Part print with two shaded views. Sizes in mm from the minimum x, y, z corner. A direction names the side the tool comes from. Give positions to 0.01 mm unless a question says otherwise; leave off trailing zeros. Write each loop counter-clockwise with the first axis right and the second up, starting at its lowest first coordinate (ties: lowest second). Pieces come first, ordered by that corner, then holes. Notation, with made-up numbers: (77.25, 6) - (120.25, 6) arc R28 cw to (120.25, 25) - close; hole circle Ø2 at (-39, 18). An arc over 180 degrees is marked (long way). Answer as a JSON object with one key per item and string values. Group by question number.
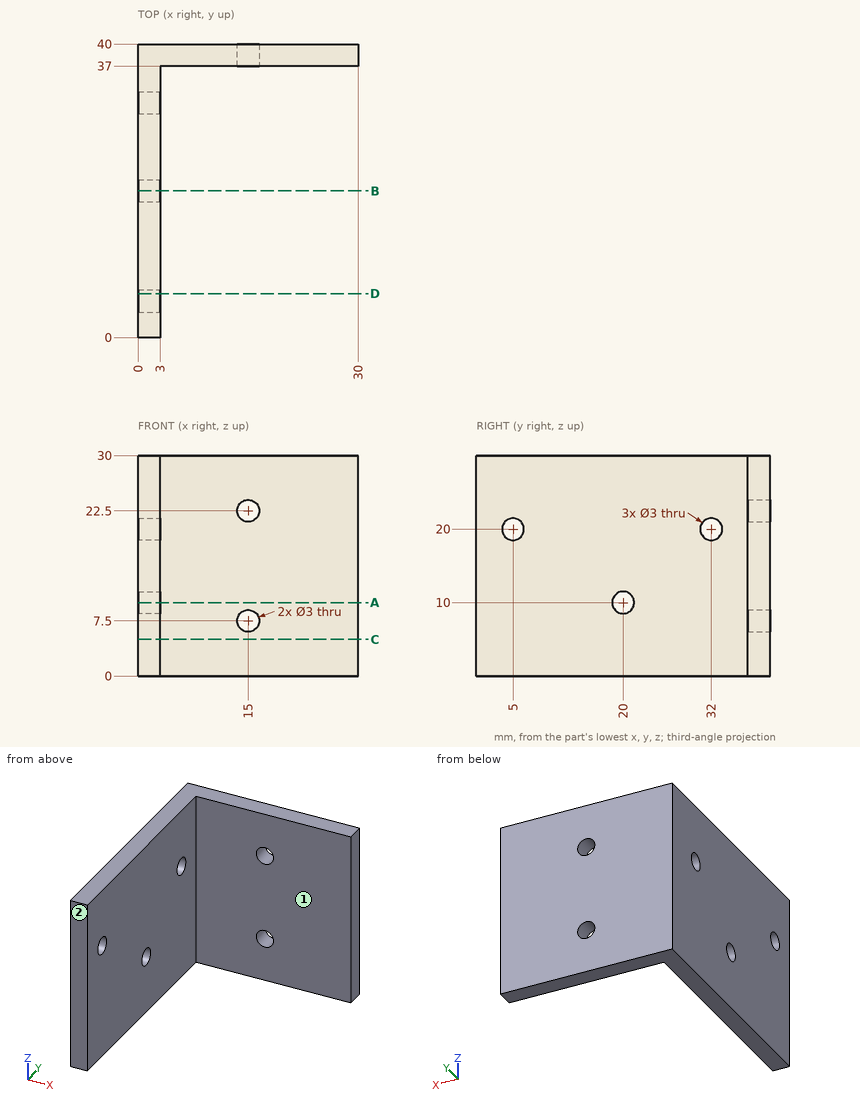
1) Drill centre lines: line 1 along Z through (x, y) = (15, 39.2); line 2 along Y through (x, z) = (2.35, 20); line 3 along X through (y, z) = (38.5, 22.5). Where is each one in solid material? Low to high. Write a range as from..to.
2) Drop flat-ended pins along their axis: P1, Ø1.8, axis at x = 15, z = 7.5, coming from the +Y side; P2, Ø1.5, axis at x = 17.5, z = 7.5, coming from the -Y side; P3, Ø1, axis at y = 26.5, z = 10, coming from the +X side. Give the stop position or say it passes through.
3) Saw through at A-A (z = 10). List the corners of the cut face in (x, y), and give its area (3 significant figures).
4) Which spindle directions (+Z, -Z, +X, -X, +Y, -Y) get a long thin tool onto all of the face, cutting with end or side? Do the marked faces 1 and 2. Say none if no direction does.
5) Saw through at D-D (y = 6). List the corners of the cut face in (x, z), and give its area (3 significant figures).
6) Saw through at C-C (z = 5). List the corners of the cut face in (x, y).
7) Saw through at B-B (y = 20). List the corners of the cut face in (x, z).
Checks:
{
 "1": {"line 1": "0..6, 9..21, 24..30", "line 2": "0..3.5, 6.5..30.5, 33.5..40", "line 3": "0..13.5, 16.5..30"},
 "2": {"P1": "through", "P2": "y = 37", "P3": "x = 3"},
 "3": {"outline": "(0, 0) - (3, 0) - (3, 18.5) - (0, 18.5) - close; (0, 21.5) - (3, 21.5) - (3, 37) - (30, 37) - (30, 40) - (0, 40) - close", "area": "192 mm2"},
 "4": {"face 1": "+Z, -Z, +X, -Y", "face 2": "+Z, -Z, +X, -X, -Y"},
 "5": {"outline": "(0, 0) - (3, 0) - (3, 18.88) - (0, 18.88) - close; (0, 21.12) - (3, 21.12) - (3, 30) - (0, 30) - close", "area": "83.3 mm2"},
 "6": {"outline": "(0, 0) - (3, 0) - (3, 37) - (30, 37) - (30, 40) - (0, 40) - close"},
 "7": {"outline": "(0, 0) - (3, 0) - (3, 8.5) - (0, 8.5) - close; (0, 11.5) - (3, 11.5) - (3, 30) - (0, 30) - close"}
}
